from build123d import *

# Parameters (mm, degrees)
CROQUIS1_W              = 37
CROQUIS1_H              = 17
SALIENTE_EXTRUIR1_DEPTH = 3.8
VACIADO1_T              = 1.8
REDONDEO2_R             = 3


with BuildPart() as part:
    # Croquis1 → Saliente-Extruir1 (new body)
    with BuildSketch(Plane(origin=(0, 0, 0), x_dir=(1, 0, 0), z_dir=(0, 1, 0))):
        Rectangle(CROQUIS1_W, CROQUIS1_H)
    extrude(amount=SALIENTE_EXTRUIR1_DEPTH)

    # Vaciado1
    vaciado1_openings = [part.faces().sort_by_distance(p)[0] for p in [
        (0, 3.8, 0),
    ]]
    offset(amount=VACIADO1_T, openings=vaciado1_openings, kind=Kind.INTERSECTION)

    # Redondeo2
    # the kernel refuses this fillet: 3 mm, written as the material it takes off along each edge
    with BuildSketch(Plane(origin=(20.3, -9.3, 10.3), x_dir=(-1, 0, 0), z_dir=(0, 1, 0)), Plane(origin=(-20.3, 11.3, 10.3), x_dir=(1, 0, 0), z_dir=(0, -1, 0)), Plane(origin=(-20.3, -9.3, -10.3), x_dir=(1, 0, 0), z_dir=(0, 1, 0)), Plane(origin=(20.3, -9.3, -10.3), x_dir=(0, 0, 1), z_dir=(0, 1, 0))) as redondeo2_piece_1:
        with BuildLine():
            CenterArc((REDONDEO2_R, -REDONDEO2_R), REDONDEO2_R, 90, 90)
            Line((0, -REDONDEO2_R), (0, 0))
            Line((0, 0), (REDONDEO2_R, 0))
        make_face()
    extrude(amount=20.6, mode=Mode.SUBTRACT)


solid = part.part
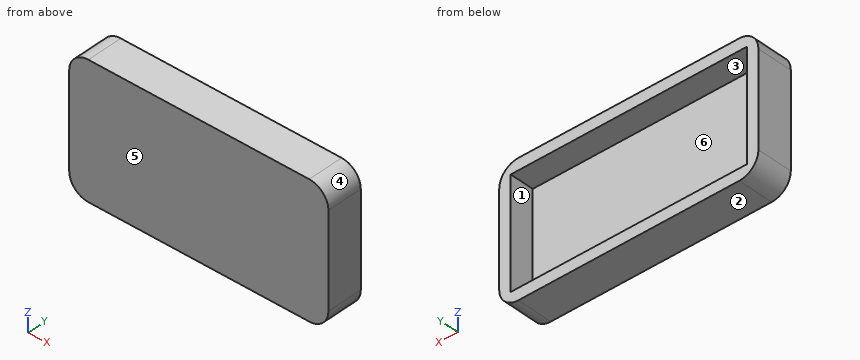
Input: part model. Units: mm. Frame: model coordinates. Face numbers are marked on the shaded views. A direction names the side the tool comes from. Round coordinates to 2 decimals unless told otherwise and drop trailing zeros. Order: outer loops, then holes, each group sorted by start corner. A loop starts at its lowest first (then second) coordinate and runs counter-clockwise, first axis right, second up. Notation, with made-up numbers: (83.5, -2) - (105.5, -2) arc R25 cw to (105.5, 17) - close; hole circle Ø1 at (38, 55.5). An arc over 180 degrees is marked (long way). Answer as a JSON object with one key per item and string values. Group by question number.
(1) Reachability of the marked faces 1 and 2 from +Z, -Z, +X, -X, +Y, -Y: full face, straight path, thin tool, end or side. Return the list, or none.
(2) Draft query along X for the marked faces 3, 4, 5 and 6. Return one class per face: released by +X, released by -X, zero draft, split by the parting line, or undercut.
(3) Material intervals for probe 1 along X at (y, z) = (2.4, 0); probe 2 along Z at (x, y) = (-4.5, 3.1); probe 3 along Y at (x, z) = (8.5, 5), sorted ascending. Write a range as from..to.
(4) Cut plane C-C (z = -0.5). Return loops of the section in (x, y), then the cut area to 3 significant figures.
(5) Cut plane B-B (x = 12). Return loops of the section in (y, z).
(6) Pin query (flat end, axial travel): P1, Ø8.5, axis at x = -4.5, z = 2.5, coming from the +Y side; P2, Ø1, axis at y = -1, z = -8, coming from the +X side. Return the tip coordinate at first contact, or that it passes through.
(7) Cut plane A-A (y = 1.9). Return loops of the section in (x, z).
Here are the results:
{
 "1": {"face 1": "+Y", "face 2": "-Z, +X, -X, +Y, -Y"},
 "2": {"face 3": "undercut", "face 4": "released by +X", "face 5": "zero draft", "face 6": "undercut"},
 "3": {"probe 1": "x = -20.3..-18.5, 18.5..20.3", "probe 2": "z = -10.3..-8.5, 8.5..10.3", "probe 3": "y = -1.8..0"},
 "4": {"outline": "(-20.3, -1.8) - (20.3, -1.8) - (20.3, 3.8) - (18.5, 3.8) - (18.5, 0) - (-18.5, 0) - (-18.5, 3.8) - (-20.3, 3.8) - close", "area": "86.8 mm^2"},
 "5": {"outline": "(-1.8, -10.3) - (3.8, -10.3) - (3.8, -8.5) - (0, -8.5) - (0, 8.5) - (3.8, 8.5) - (3.8, 10.3) - (-1.8, 10.3) - close"},
 "6": {"P1": "stops at y = 0", "P2": "stops at x = 20.29"},
 "7": {"outline": "(-20.3, -7.3) arc R3 ccw to (-17.3, -10.3) - (17.3, -10.3) arc R3 ccw to (20.3, -7.3) - (20.3, 7.3) arc R3 ccw to (17.3, 10.3) - (-17.3, 10.3) arc R3 ccw to (-20.3, 7.3) - close; hole (-18.5, -8.5) - (18.5, -8.5) - (18.5, 8.5) - (-18.5, 8.5) - close"}
}
